from build123d import *

# Parameters (mm, degrees)
ESQUISSE2_W             = 95.08
ESQUISSE2_H             = 114.3
ESQUISSE2_R             = 1
ESQUISSE2_W_2           = 22.362765252
ESQUISSE2_H_2           = 29.888087148
ESQUISSE2_W_3           = 9.312830524
ESQUISSE2_H_3           = 18
ESQUISSE2_W_4           = 28.571334831
ESQUISSE2_H_4           = 18.895330988
ESQUISSE2_W_5           = 3
ESQUISSE2_H_5           = 6
BOSS_EXTRU_1_DEPTH      = 4
CONG_1_R                = 3
ESQUISSE3_R             = 1
ENL_V_MAT_EXTRU_1_DEPTH = 10
ENL_V_START             = -10
ESQUISSE4_R             = 1
ENL_V_MAT_EXTRU_2_DEPTH = 10
CONG_2_R                = 3


with BuildPart() as part:
    # Esquisse2 → Boss.-Extru.1 (new body)
    with BuildSketch(Plane.XY):
        Rectangle(ESQUISSE2_W, ESQUISSE2_H)
        with Locations((-33.669054573, -42.15)):
            Circle(ESQUISSE2_R, mode=Mode.SUBTRACT)
        with Locations((5.450945427, -42.15)):
            Circle(ESQUISSE2_R, mode=Mode.SUBTRACT)
        with Locations((5.450945427, -24.15)):
            Circle(ESQUISSE2_R, mode=Mode.SUBTRACT)
        with Locations((-33.669054573, -24.15)):
            Circle(ESQUISSE2_R, mode=Mode.SUBTRACT)
        with Locations(Location((-33.669054573, 24.15, 0), (0, 0, 180))):
            Circle(ESQUISSE2_R, mode=Mode.SUBTRACT)
        with Locations(Location((5.450945427, 24.15, 0), (0, 0, 180))):
            Circle(ESQUISSE2_R, mode=Mode.SUBTRACT)
        with Locations(Location((5.450945427, 42.15, 0), (0, 0, 180))):
            Circle(ESQUISSE2_R, mode=Mode.SUBTRACT)
        with Locations(Location((-33.669054573, 42.15, 0), (0, 0, 180))):
            Circle(ESQUISSE2_R, mode=Mode.SUBTRACT)
        with Locations((24.358617374, 29.442657314)):
            Rectangle(ESQUISSE2_W_2, ESQUISSE2_H_2, mode=Mode.SUBTRACT)
        with Locations((-14.585732185, 33.15)):
            Rectangle(ESQUISSE2_W_3, ESQUISSE2_H_3, mode=Mode.SUBTRACT)
        with Locations((-14.585732185, -33.15)):
            Rectangle(ESQUISSE2_W_3, ESQUISSE2_H_3, mode=Mode.SUBTRACT)
        with Locations((-21.254332584, 0)):
            Rectangle(ESQUISSE2_W_4, ESQUISSE2_H_4, mode=Mode.SUBTRACT)
        with Locations((24.358617374, -29.442657314)):
            Rectangle(ESQUISSE2_W_2, ESQUISSE2_H_2, mode=Mode.SUBTRACT)
        with Locations((41.54, 0)):
            Rectangle(ESQUISSE2_W_5, ESQUISSE2_H_5, mode=Mode.SUBTRACT)
        with Locations((41.54, -50)):
            Rectangle(ESQUISSE2_W_5, ESQUISSE2_H_5, mode=Mode.SUBTRACT)
        with Locations((41.54, 50)):
            Rectangle(ESQUISSE2_W_5, ESQUISSE2_H_5, mode=Mode.SUBTRACT)
        with Locations((-41.54, 50)):
            Rectangle(ESQUISSE2_W_5, ESQUISSE2_H_5, mode=Mode.SUBTRACT)
        with Locations((-41.54, 0)):
            Rectangle(ESQUISSE2_W_5, ESQUISSE2_H_5, mode=Mode.SUBTRACT)
        with Locations((-41.54, -50)):
            Rectangle(ESQUISSE2_W_5, ESQUISSE2_H_5, mode=Mode.SUBTRACT)
    extrude(amount=BOSS_EXTRU_1_DEPTH)

    # Congé1
    cong_1_edges = [part.edges().sort_by_distance(p)[0] for p in [
        (-9.929316923, 24.15, 2),
        (-9.929316923, 42.15, 2),
        (-19.242147447, 42.15, 2),
        (-19.242147447, 24.15, 2),
        (-9.929316923, -42.15, 2),
        (-9.929316923, -24.15, 2),
        (-19.242147447, -24.15, 2),
        (-19.242147447, -42.15, 2),
        (-35.54, 9.447665494, 2),
        (-35.54, -9.447665494, 2),
        (-6.968665169, -9.447665494, 2),
        (-6.968665169, 9.447665494, 2),
        (35.54, -44.386700888, 2),
        (35.54, -14.49861374, 2),
        (13.177234748, -14.49861374, 2),
        (13.177234748, -44.386700888, 2),
        (35.54, 14.49861374, 2),
        (35.54, 44.386700888, 2),
        (13.177234748, 44.386700888, 2),
        (13.177234748, 14.49861374, 2),
    ]]
    fillet(cong_1_edges, radius=CONG_1_R)

    # Esquisse3 → Enlèv. mat.-Extru.1 (cut)
    with BuildSketch(Plane(origin=(47.54, 0, 0), x_dir=(0, 0, -1), z_dir=(1, 0, 0))):
        with Locations(Location((-2, 50, 0), (0, 0, 90))):
            Circle(ESQUISSE3_R)
        with Locations(Location((-2, 0, 0), (0, 0, 90))):
            Circle(ESQUISSE3_R)
        with Locations(Location((-2, -50, 0), (0, 0, 90))):
            Circle(ESQUISSE3_R)
    extrude(amount=-ENL_V_MAT_EXTRU_1_DEPTH, mode=Mode.SUBTRACT)

    # Esquisse4 → Enlèv. mat.-Extru.2 (cut)
    with BuildSketch(Plane.ZY.offset(47.54).offset(ENL_V_START)):
        with Locations(Location((2, 50, 0), (0, 0, 90))):
            Circle(ESQUISSE4_R)
        with Locations(Location((2, 0, 0), (0, 0, 90))):
            Circle(ESQUISSE4_R)
        with Locations(Location((2, -50, 0), (0, 0, 90))):
            Circle(ESQUISSE4_R)
    extrude(amount=ENL_V_MAT_EXTRU_2_DEPTH, mode=Mode.SUBTRACT)

    # Congé2
    cong_2_edges = [part.edges().sort_by_distance(p)[0] for p in [
        (0, -57.15, 4),
        (0, 57.15, 4),
    ]]
    fillet(cong_2_edges, radius=CONG_2_R)


solid = part.part
Work out the finished part from the listing and answer in its coordinate system (mm). Round coordinates to 2 decimals unless told otherwise and drop trailing zeros. Write each loop counter-clockwise with the first axis right and the second up, starting at its lowest first coordinate (ties: lowest second). Pieces come first, ordered by that corner, then holes. Notation, with made-up numbers: (40, 65) -> (47, 65) arc R14 ccw to (47, 85) -> close; hole circle Ø2 at (-19, 72). An arc over 180 degrees is marked (long way). Answer as CSV lines item,"result". Start each with the question number.
(1) The part is cut by section B-B, the plane x = -27. Give the vertices of the cut face in (y, z).
(2) The part is cut by section D-D, the plane z = 2. Give the number of separate pieces and of enclosed holes in the cut face, then the cut area to 3 significant figures.
(3) Find the intervals of material crossed by probe 1 along X at (y, z) = (38, 1.75); probe 2 along X at (y, z) = (-1.5, 0.5); probe 3 along X at (y, z) = (21, 2.6), in increasing order.
(4) The part is cut by section C-C, the plane y = -29. Give the vertices of the cut face in (x, z), then the cut area to 3 significant figures.
(5) The part is cut by section A-A, the plane x = 29. Give the vertices of the cut face in (y, z).
(6) The mould has two halves that part along Y. Classify faces 1 (the flat face through (40.04, 1, 3)), 2 (the flat face through (-1, 1, 4)): +Y half, -Y half, draft (parallel to the pull), parting line (faces both ways), or undercut.
(7) Each of these flat-tipped pins is pushed along its axis until it touches: pin 1 (1.2 mm diameter, centred on y = -50, z = 2, fed in from -X); pin 2 (0.9 mm diameter, centred on x = -41.5, z = 2.5, fed in from -Y); pin 3 (1 mm diameter, centred on x = -4.5, z = 3, fed in from +Y). Where does it stop, or does it pass through?
Output values:
1,outline,"(-57.15, 0) -> (-9.45, 0) -> (-9.45, 4) -> (-54.15, 4) arc R3 ccw to (-57.15, 1) -> close; (9.45, 0) -> (57.15, 0) -> (57.15, 1) arc R3 ccw to (54.15, 4) -> (9.45, 4) -> close"
2,separate pieces,"1"
2,enclosed holes,"13"
2,area,"8,440 mm²"
3,probe 1,"x = -47.54 to -19.24, -9.93 to 13.18, 35.54 to 47.54"
3,probe 2,"x = -47.54 to -43.04, -40.04 to -35.54, -6.97 to 40.04, 43.04 to 47.54"
3,probe 3,"x = -47.54 to 13.18, 35.54 to 47.54"
4,outline,"(-47.54, 0) -> (-19.24, 0) -> (-19.24, 4) -> (-47.54, 4) -> close; (-9.93, 0) -> (13.18, 0) -> (13.18, 4) -> (-9.93, 4) -> close; (35.54, 0) -> (47.54, 0) -> (47.54, 4) -> (35.54, 4) -> close"
4,area,"254 mm²"
5,outline,"(-57.15, 0) -> (-44.39, 0) -> (-44.39, 4) -> (-54.15, 4) arc R3 ccw to (-57.15, 1) -> close; (-14.5, 0) -> (14.5, 0) -> (14.5, 4) -> (-14.5, 4) -> close; (44.39, 0) -> (57.15, 0) -> (57.15, 1) arc R3 ccw to (54.15, 4) -> (44.39, 4) -> close"
6,face 1,"undercut"
6,face 2,"draft"
7,pin 1,"stops at x = -37.54"
7,pin 2,"stops at y = -56.96"
7,pin 3,"stops at y = 56.75"
